```python
from build123d import *

# Parameters (mm, degrees)
RECTANGULAR_TUBE_CONFIGURED_60_X_40_X_DEPTH = 680


with BuildPart() as part:
    # Sketch1 → Rectangular tube - configured 60 X 40 X 3.2(2) (new body)
    with BuildSketch(Plane.YZ.offset(-340)):
        with BuildLine():
            Line((-13.6, -30), (13.6, -30))
            ThreePointArc((13.6, -30), (18.1254834, -28.1254834), (20, -23.6))
            Line((20, -23.6), (20, 23.6))
            ThreePointArc((20, 23.6), (18.1254834, 28.1254834), (13.6, 30))
            Line((13.6, 30), (-13.6, 30))
            ThreePointArc((-13.6, 30), (-18.1254834, 28.1254834), (-20, 23.6))
            Line((-20, 23.6), (-20, -23.6))
            ThreePointArc((-20, -23.6), (-18.1254834, -28.1254834), (-13.6, -30))
        make_face()
        with BuildLine():
            Line((-13.6, -27), (13.6, -27))
            ThreePointArc((13.6, -27), (16.004163056, -26.004163056), (17, -23.6))
            Line((17, -23.6), (17, 23.6))
            ThreePointArc((17, 23.6), (16.004163056, 26.004163056), (13.6, 27))
            Line((13.6, 27), (-13.6, 27))
            ThreePointArc((-13.6, 27), (-16.004163056, 26.004163056), (-17, 23.6))
            Line((-17, 23.6), (-17, -23.6))
            ThreePointArc((-17, -23.6), (-16.004163056, -26.004163056), (-13.6, -27))
        make_face(mode=Mode.SUBTRACT)
    extrude(amount=RECTANGULAR_TUBE_CONFIGURED_60_X_40_X_DEPTH)


solid = part.part
```
Input: part model. Units: mm. Frame: model coordinates. A direction names the side the tool comes from. Coordinates: 2 decimals unless noted, no trailing zeros. Loops run counter-clockwise (first coordinate to the right, second up) from the corner with the lowest first, then second, coordinate; pieces in that order, holes last. Notation, with made-up numbers: (35.5, 27) - (47.5, 27) arc R14 cw to (47.5, 46) - close; hole circle Ø11 at (-3, 35.25). An arc over 180 degrees is marked (long way). Answer in a Markdown table with one row per item.
(1) Cut plane B-B on z = -13.5. Output: boundary loops of the cut face in (x, y), plus the area to 3 significant figures.
Model answer:
| item | result |
|---|---|
| outline | (-340, -20) - (340, -20) - (340, -17) - (-340, -17) - close; (-340, 17) - (340, 17) - (340, 20) - (-340, 20) - close |
| area | 4,080 mm² |
(2) Set-up query: faces 1 (the face through (-5, 0, 30)), 2 (the face through (-5, -17, 0)). Return all of +Z, -Z, +X, -X, +Y, -Y with unobstructed straight access to the full face (end or side cutting, diameter ignored); none if empty.
Model answer:
| item | result |
|---|---|
| face 1 | +Z, +X, -X, +Y, -Y |
| face 2 | +X, -X |
(3) Mould query, pull axis Z, two halves, no side actions, for faces 3 (the face through (340, -18, -2)), 4 (the face through (-5, 0, -30)), 5 (the face through (-5, 0, -27)). Classes: pulls with the +Z half, pulls with the -Z half, needs draft (parallel to the pull), parting line crosses it, or undercut.
Model answer:
| item | result |
|---|---|
| face 3 | needs draft |
| face 4 | pulls with the -Z half |
| face 5 | undercut |
(4) Cut plane C-C on y = -1. Output: boundary loops of the cut face in (x, z), plus the area to 3 significant figures.
Model answer:
| item | result |
|---|---|
| outline | (-340, -30) - (340, -30) - (340, -27) - (-340, -27) - close; (-340, 27) - (340, 27) - (340, 30) - (-340, 30) - close |
| area | 4,080 mm² |
(5) Cut plane A-A on x = -86. Output: boundary loops of the cut face in (y, z).
Model answer:
| item | result |
|---|---|
| outline | (-20, -23.6) arc R6.4 ccw to (-13.6, -30) - (13.6, -30) arc R6.4 ccw to (20, -23.6) - (20, 23.6) arc R6.4 ccw to (13.6, 30) - (-13.6, 30) arc R6.4 ccw to (-20, 23.6) - close; hole (-17, -23.6) arc R3.4 ccw to (-13.6, -27) - (13.6, -27) arc R3.4 ccw to (17, -23.6) - (17, 23.6) arc R3.4 ccw to (13.6, 27) - (-13.6, 27) arc R3.4 ccw to (-17, 23.6) - close |
(6) Material intervals for L1, parallel to Y at x = 188, z = -3; L2, parallel to Z at x = -103, y = 10.5; L3, parallel to Z at x = 166, y = 15 (3 decimals), sorted ascending. Write a range as from..to.
Model answer:
| item | result |
|---|---|
| L1 | y = -20..-17, 17..20 |
| L2 | z = -30..-27, 27..30 |
| L3 | z = -29.845..-26.698, 26.698..29.845 |
